Design review of the part built by this model. Coordinates are the model's own, in mm. Face numbers are marked on the shaded views. A direction names the side the tool comes from. Give positions to 0.01 mm unless a question says otherwise; leave off trailing zeros. Write each loop counter-clockwise with the first axis right and the second up, starting at its lowest first coordinate (ties: lowest second). Pieces come first, ordered by that corner, then holes. Notation, with made-up numbers: (20.25, 23.25) - (50.25, 23.25) arc R11 cw to (50.25, 36.25) - close; hole circle Ø10 at (49.5, 26.25). An arc over 180 degrees is marked (long way). Use a Markdown table: item, result. Add a question column.
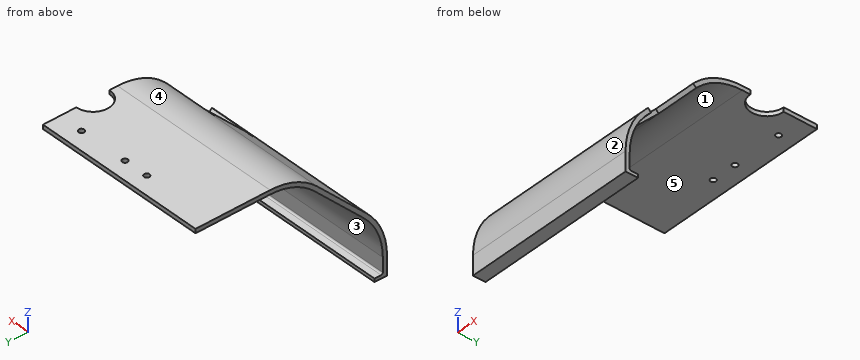
```python
from build123d import *

# Parameters (mm, degrees)
PAD_DEPTH            = 105
PAD_DEPTH_BACK       = 105
SKETCH001_R          = 1.65
SKETCH001_W          = 38.25
SKETCH001_H          = 51.5
POCKET_DEPTH         = 101.705966
SKETCH003_R          = 1.65
POCKET001_DEPTH      = 5
SKETCH004_W          = 2
SKETCH004_H          = 210
PAD001_DEPTH         = 5
FILLET_R             = 1
SKETCH005_R          = 10
POCKET002_DEPTH      = 5
SKETCH006_W          = 110
SKETCH006_H          = 90
POCKET003_DEPTH      = 100
POCKET003_DEPTH_BACK = -72


with BuildPart() as part:
    # Sketch → Pad (new body, two sides)
    with BuildSketch(Plane.YZ) as pad_sk:
        with BuildLine():
            Line((12.736792, 82.5), (57.500792, 82.5))
            Line((57.500792, 82.5), (57.500792, 80))
            Line((57.500792, 80), (12.736792, 80))
            ThreePointArc((12.736792, 80), (-1.613837, 77.145482), (-13.779712, 69.016504))
            Line((-13.779712, 69.016504), (-43.478197, 39.318019))
            ThreePointArc((-43.478197, 39.318019), (-52.006167, 26.55501), (-55.000792, 11.500014))
            Line((-55.000792, 11.500014), (-55.000792, 0))
            Line((-55.000792, 0), (-57.500792, 0))
            Line((-57.500792, 11.500014), (-57.500792, 0))
            ThreePointArc((-45.245964, 41.085786), (-54.315866, 27.511719), (-57.500792, 11.500014))
            Line((-15.547479, 70.784271), (-45.245964, 41.085786))
            ThreePointArc((12.736792, 82.5), (-2.570545, 79.455181), (-15.547479, 70.784271))
        make_face()
    extrude(amount=PAD_DEPTH)
    extrude(pad_sk.sketch, amount=-PAD_DEPTH_BACK)

    # Sketch001 (on Face12 of Pad) → Pocket (cut, through all)
    with BuildSketch(Plane(origin=(0, -43.165875, 43.165875), x_dir=(0, -0.707107, -0.707107), z_dir=(0, -0.707107, 0.707107))):
        with Locations((-34.55831, 28.7)):
            Circle(SKETCH001_R)
        with Locations((-1.55831, 28.7)):
            Circle(SKETCH001_R)
        with Locations((-34.55831, -28.7)):
            Circle(SKETCH001_R)
        with Locations((-1.55831, -28.7)):
            Circle(SKETCH001_R)
        with Locations((-18.05831, 0)):
            Rectangle(SKETCH001_W, SKETCH001_H)
    extrude(amount=-POCKET_DEPTH, mode=Mode.SUBTRACT)

    # Sketch003 (on Face2 of Pocket) → Pocket001 (cut)
    with BuildSketch(Plane(origin=(0, 0, 82.5), x_dir=(0, -1, 0), z_dir=(0, 0, 1))):
        with Locations((-47.500792, 15)):
            Circle(SKETCH003_R)
        with Locations((-47.500792, 45)):
            Circle(SKETCH003_R)
        with Locations((-47.500792, -15)):
            Circle(SKETCH003_R)
        with Locations((-47.500792, -45)):
            Circle(SKETCH003_R)
        with Locations((-47.500792, 60)):
            Circle(SKETCH003_R)
        with Locations((-47.500792, -60)):
            Circle(SKETCH003_R)
    extrude(amount=-POCKET001_DEPTH, mode=Mode.SUBTRACT)

    # Sketch004 (on Face26 of Pocket001) → Pad001 (join)
    with BuildSketch(Plane.ZX.offset(-55.000792)):
        with Locations((1, 0)):
            Rectangle(SKETCH004_W, SKETCH004_H)
    extrude(amount=PAD001_DEPTH)

    # Fillet
    fillet_edges = [part.edges().sort_by_distance(p)[0] for p in [
        (0, -55.000792, 2),
    ]]
    fillet(fillet_edges, radius=FILLET_R)

    # Sketch005 (on Face15 of Fillet) → Pocket002 (cut)
    with BuildSketch(Plane(origin=(0, 0, 82.5), x_dir=(0, -1, 0), z_dir=(0, 0, 1))):
        with Locations((-27.500792, 0)):
            Circle(SKETCH005_R)
    extrude(amount=-POCKET002_DEPTH, mode=Mode.SUBTRACT)

    # Sketch006 → Pocket003 (cut, two sides)
    with BuildSketch(Plane.XZ) as pocket003_sk:
        with Locations((55, 45)):
            Rectangle(SKETCH006_W, SKETCH006_H)
    extrude(amount=-POCKET003_DEPTH, mode=Mode.SUBTRACT)
    extrude(pocket003_sk.sketch, amount=-POCKET003_DEPTH_BACK, mode=Mode.SUBTRACT)


solid = part.part
```
(1) Add section C-C (x = -72). State the section outline as (y, z) points, and give its area (3 significant figures).
(2) Insertion check: pin 1 (2 mm diameter, centred on x = -45, y = 47.5, fed in from -Z); pin 2 (7 mm diameter, centred on x = -31, z = 8.5, fed in from +Y); pin 3 (2 mm diameter, centred on x = -56, z = 0.5, fed in from +Y); pin 4 (2 mm diameter, centred on x = -41, y = -51.5, fed in from +Z). Each pin has a flat end and moves straight along its axis. Give the tip position at first contact, or say it passes through.
(3) Add section B-B (x = -15). State the section outline as (y, z) points.
(4) Mouldability with a two-part tool opening along Z and no side actions: class the marked faces 1, 2 and 3 as +Z half, -Z half, draft (parallel to the pull), parting line (faces both ways), or undercut.
(5) For line 1 along Z through (x, y) = (-8, 42.5); line 2 along Z through (x, y) = (-72, -52); line 3 along Y through (x, z) = (-57.5, 51.5), list the stretches that pass through material, from the lowest coordinate up.
(6) Tool access review of the marked faces 4 and 5: name each direction out of +Z, -Z, +X, -X, +Y, -Y from which nothing blocks a thin tool from reaching the whole face with its end or side.
(7) Add section A-A (x = -60). State the section outline as (y, z) points.
(8) Add section D-D (y = 2.5). State the section outline as (x, z) points, and give its area (3 significant figures).
Answers follow:
| question | item | result |
|---|---|---|
| 1 | outline | (-57.5, 0) - (-50, 0) - (-50, 2) - (-54, 2) arc R1 cw to (-55, 3) - (-55, 11.5) arc R39.34 cw to (-43.48, 39.32) - (-13.78, 69.02) arc R37.5 cw to (12.74, 80) - (57.5, 80) - (57.5, 82.5) - (12.74, 82.5) arc R40 ccw to (-15.55, 70.78) - (-45.25, 41.09) arc R41.84 ccw to (-57.5, 11.5) - close |
| 1 | area | 412 mm^2 |
| 2 | pin 1 | through |
| 2 | pin 2 | y = -55 |
| 2 | pin 3 | y = -50 |
| 2 | pin 4 | z = 34.67 |
| 3 | outline | (-57.5, 0) - (-50, 0) - (-50, 2) - (-54, 2) arc R1 cw to (-55, 3) - (-55, 11.5) arc R39.34 cw to (-43.48, 39.32) - (-42.15, 40.64) - (-43.92, 42.41) - (-45.25, 41.09) arc R41.84 ccw to (-57.5, 11.5) - close; (-16.87, 69.46) - (-15.11, 67.69) - (-13.78, 69.02) arc R37.5 cw to (12.74, 80) - (45.85, 80) - (45.85, 82.5) - (12.74, 82.5) arc R40 ccw to (-15.55, 70.78) - close; (49.15, 80) - (57.5, 80) - (57.5, 82.5) - (49.15, 82.5) - close |
| 4 | face 1 | -Z half |
| 4 | face 2 | +Z half |
| 4 | face 3 | undercut |
| 5 | line 1 | 80 to 82.5 |
| 5 | line 2 | 0 to 2, 26.57 to 32.24 |
| 5 | line 3 | -34.83 to -31.3 |
| 6 | face 4 | +Z, +X, -X, -Y |
| 6 | face 5 | -Z, +X, -X, +Y |
| 7 | outline | (-57.5, 0) - (-50, 0) - (-50, 2) - (-54, 2) arc R1 cw to (-55, 3) - (-55, 11.5) arc R39.34 cw to (-43.48, 39.32) - (-13.78, 69.02) arc R37.5 cw to (12.74, 80) - (45.85, 80) - (45.85, 82.5) - (12.74, 82.5) arc R40 ccw to (-15.55, 70.78) - (-45.25, 41.09) arc R41.84 ccw to (-57.5, 11.5) - close; (49.15, 80) - (57.5, 80) - (57.5, 82.5) - (49.15, 82.5) - close |
| 8 | outline | (-105, 78.58) - (0, 78.58) - (0, 81.17) - (-105, 81.17) - close |
| 8 | area | 272 mm^2 |
